from build123d import *

# Parameters (mm, degrees)
BOSS_EXTRUDE1_DEPTH = 1.905
SKETCH2_R           = 0.254
BOSS_EXTRUDE2_DEPTH = 25.4


with BuildPart() as part:
    # Sketch1 → Boss-Extrude1 (new body)
    with BuildSketch(Plane(origin=(0, 0, 0), x_dir=(1, 0, 0), z_dir=(0, 1, 0))):
        with BuildLine():
            Line((-1.397, 2.1844), (1.397, 2.1844))
            ThreePointArc((1.397, 2.1844), (2.54, 0), (1.397, -2.1844))
            Line((1.397, -2.1844), (-1.397, -2.1844))
            ThreePointArc((-1.397, -2.1844), (-2.54, 0), (-1.397, 2.1844))
        make_face()
    extrude(amount=BOSS_EXTRUDE1_DEPTH)

    # Sketch2 → Boss-Extrude2 (add)
    with BuildSketch(Plane.XZ):
        with Locations(Location((-1.651, 0, 0), (0, 0, 90))):
            Circle(SKETCH2_R)
        with Locations(Location((1.651, 0, 0), (0, 0, 90))):
            Circle(SKETCH2_R)
    extrude(amount=BOSS_EXTRUDE2_DEPTH)


solid = part.part
Build history of the part. All positions in model axes, mm. Round coordinates to 2 decimals unless told otherwise and drop trailing zeros. Order: outer loops, then holes, each group sorted by start corner. A loop starts at its lowest first (then second) coordinate and runs counter-clockwise, first axis right, second up. Notation, with made-up numbers: M 16,49 L 55,49 A30 cw 55,78 Z; hole C 26.25,66.5 d7. An arc over 180 degrees is marked long. Use CSV: the item, a comma, the result in double quotes. Start each with the question number.
(1) Cut at D-D on y = -15.5. List the corners of the cut face in (x, z), then the cut area to 3 significant figures.
(2) Flat gauge pin, fed straight in: P1, Ø2, axis at y = -14, z = -0.5, coming from the +X side (3 decimals). Where does the tip first touch, or does it go through?
(3) Drill centre lines: probe 1 along X at (y, z) = (-19.5, -0.2); probe 2 along Y at (x, z) = (0.85, -1.15) (3 decimals); probe 3 along Z at (x, y) = (1.6, -4.25). Where is each one in solid material? Low to high.
(4) Cut at A-A on z = 0. List the corners of the cut face in (x, y) (3 decimals), then the cut area to 3 significant figures.
(5) Cut at B-B on y = 0.25. List the corners of the cut face in (x, z), then the cut area to 3 significant figures.
(6) Cut at C-C on x = 1.05. List the corners of the cut face in (y, z) (3 decimals).
Findings:
1,outline,"C -1.65,0 d0.51; C 1.65,0 d0.51"
1,area,"0.405 mm^2"
2,P1,"stops at x = 1.905"
3,probe 1,"x = -1.81 to -1.49, 1.49 to 1.81"
3,probe 2,"y = 0 to 1.905"
3,probe 3,"z = -0.25 to 0.25"
4,outline,"M -2.54,0 L -1.905,0 L -1.905,-25.4 L -1.397,-25.4 L -1.397,0 L 1.397,0 L 1.397,-25.4 L 1.905,-25.4 L 1.905,0 L 2.54,0 L 2.54,1.905 L -2.54,1.905 Z"
4,area,"35.5 mm^2"
5,outline,"M -1.4,-2.18 L 1.4,-2.18 A2.66 ccw 1.4,2.18 L -1.4,2.18 A2.66 ccw Z"
5,area,"19.2 mm^2"
6,outline,"M 0,-2.184 L 1.905,-2.184 L 1.905,2.184 L 0,2.184 Z"
